Autodesk Inventor part; units mm, degrees
ref_plane "YZ Plane" through (0, 0, 0) normal (1, 0, 0) x (0, 1, 0)
ref_plane "XZ Plane" through (0, 0, 0) normal (0, 1, 0) x (-1, 0, 0)
ref_plane "XY Plane" through (0, 0, 0) normal (0, 0, 1) x (1, 0, 0)
sketch "Esquisse1" plane through (0, 0, 0) normal (1, 0, 0) x (0, 1, 0)
  line L0 (10, 13.8) -> (-32, 13.8)
  line L1 (-32, 13.8) -> (-32, -7)
  line L2 (-32, -7) -> (10, -7)
  line L3 (10, -7) -> (10, 13.8)
  point P0 (0, 0)
  dimension "d0" = 42
  dimension "d1" = 20.8
extrude "Extrusion1" add sketch "Esquisse1" along normal blind 40
sketch "Esquisse2" plane through (40, 0, 0) normal (1, 0, 0) x (0, 0, -1)
  circle A0 centre (-3, 0) radius 4
  line L0 (7, 10) -> (-13.8, 10)
  line L1 (-3.4, 0) -> (-13.8, 0)
  line L2 (-3, 0) -> (7, 0)
  point P0 (0, 0)
  dimension "d4" = 10
extrude "Extrusion2" add sketch "Esquisse2" along normal blind 10
fillet "Congé1" radius 3 8 edges at (20, 10, 13.8) (20, 10, -7) (0, 10, 3.4) (0, -11, 13.8) (0, -11, -7) (0, -32, 3.4) (20, -32, 13.8) (20, -32, -7)
properties part number "servomoteur"
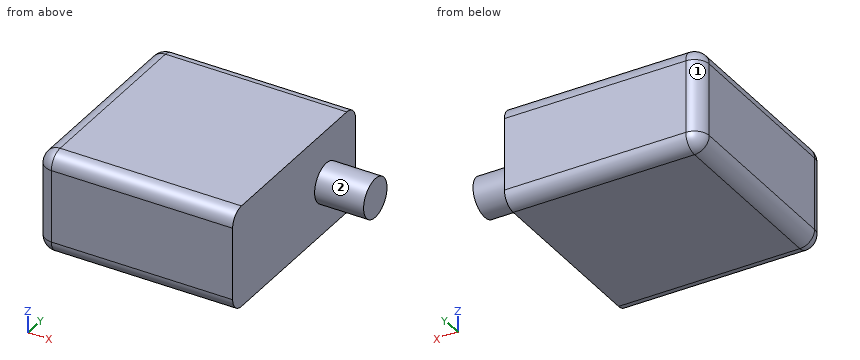
Source: CAD feature listing. Evaluate the final solid. Frame: model axes, mm. Face numbers are marked on the shaded views. A direction names the side the tool comes from. Round coordinates to 2 decimals unless told otherwise and drop trailing zeros. Loops run counter-clockwise (first coordinate to the right, second up) from the corner with the lowest first, then second, coordinate; pieces in that order, holes last.
(1) Section query D-D (y = 6). Output: boundary loops of the cut face in (x, z).
From the geometry:
outline: (0, -4) arc R3 ccw to (3, -7) - (40, -7) - (40, 13.8) - (3, 13.8) arc R3 ccw to (0, 10.8) - close
(2) Contact query for flat-ended pins moving along their axis: pin 1 Ø5 at (x, z) = (43, -3) entering from +Y; pin 2 Ø10 at (y, z) = (-23.5, -2.5) entering from +X. Output: stop coordinate, or through.
From the geometry:
pin 1: stops at y = 1.94
pin 2: stops at x = 40
(3) Section query A-A (y = 0). Output: boundary loops of the cut face in (x, z).
From the geometry:
outline: (0, -4) arc R3 ccw to (3, -7) - (40, -7) - (40, -1) - (50, -1) - (50, 7) - (40, 7) - (40, 13.8) - (3, 13.8) arc R3 ccw to (0, 10.8) - close
(4) Material intervals for probe 1 along X at (y, z) = (3.5, 5.5); probe 2 along Y at (x, z) = (30, 12); probe 3 along X at (y, z) = (-23, -5), sorted ascending.
From the geometry:
probe 1: x = 0 to 40
probe 2: y = -31.75 to 9.75
probe 3: x = 0.17 to 40
(5) Section query B-B (z = 5). Output: boundary loops of the cut face in (x, y).
From the geometry:
outline: (0, -29) arc R3 ccw to (3, -32) - (40, -32) - (40, -3.46) - (50, -3.46) - (50, 3.46) - (40, 3.46) - (40, 10) - (3, 10) arc R3 ccw to (0, 7) - close
(6) Access query for the marked faces 1 and 2. Directions: +Z, -Z, +X, -X, +Y, -Y. A direction counts if a zero-diameter tool reaches every point of the face in a straight line with its end or side. Return the directions, or none.
From the geometry:
face 1: +Z, -Z, -X, +Y
face 2: +X
(7) Section query C-C (x = 43). Output: boundary loops of the cut face in (y, z), and give its area (3 significant figures).
From the geometry:
outline: circle Ø8 at (0, 3)
area: 50.3 mm2
